Check sheet for the modelled part. Datum: model origin and axes. Units: mm. A direction names the side the tool comes from. Coordinates: 2 decimals unless noted, no trailing zeros. Loops run counter-clockwise (first coordinate to the right, second up) from the corner with the lowest first, then second, coordinate; pieces in that order, holes last. Notation, with made-up numbers: M 38,82 L 78,82 A16 ccw 78,93 Z; hole C 71,-36 d11. An arc over 180 degrees is marked long. Answer as CSV lines item,"result". Start each with the question number.
from build123d import *

# Parameters (mm, degrees)
F1_DEPTH = 15
F2_R     = 10
F3_R     = 5
F4_R     = 5


with BuildPart() as f1:
    # F0 (on Front) → F1 (new body)
    with BuildSketch(Plane.XZ):
        Polygon((41.584589, 20), (41.584589, 0), (48.584589, 0), (48.584589, 27), (19.284589, 27), (19.284589, 7), (-45.715411, 7), (-50.715411, 7), (-50.715411, 0), (26.284589, 0), (26.284589, 20), align=None)
    extrude(amount=F1_DEPTH)

    # F2
    f2_edges = [f1.edges().sort_by_distance(p)[0] for p in [
        (19.284589, -7.5, 7),
    ]]
    fillet(f2_edges, radius=F2_R)

    # F3
    f3_edges = [f1.edges().sort_by_distance(p)[0] for p in [
        (19.284589, -7.5, 27),
    ]]
    fillet(f3_edges, radius=F3_R)

    # F4
    f4_edges = [f1.edges().sort_by_distance(p)[0] for p in [
        (48.584589, -7.5, 27),
    ]]
    fillet(f4_edges, radius=F4_R)


solid = f1.part
Item 1: Go/stop test with flat-tipped pins: pin 1 (4.5 mm diameter, centred on x = -34.5, y = -11, fed in from +Z); pin 2 (1.5 mm diameter, centred on y = -7, z = 19, fed in from -X); pin 3 (7.5 mm diameter, centred on x = 34, y = -8, fed in from -Z). Record where each tip stops, or that it passes through.
Item 2: Sectioned sample at B-B, the plane y = -9. Record the boundary of the cut face in (x, z), and give its area (3 significant figures).
Item 3: Sectioned sample at A-A, the plane z = 4. Record the boundary of the cut face in (x, y).
Item 4: Sectioned sample at C-C, the plane z = 11.5. Record the boundary of the cut face in (x, y), and give its area (3 significant figures).
Item 5: Material ranges on line 1 (X direction, y = -12, z = 2.25); line 2 (X direction, y = -13.75, z = 18.5); line 3 (X direction, y = -6.25, z = 22.25), recorded low to high. Write a range as from..to.
Item 6: Release check for a two-part mould opening along X. For faces 1 (the face through (26.285, -7, 10)), 2 (the face through (34, -7, 27)), 3 (the face through (-50.715, -7, 4)), 4 (the face through (34, -7, 20)) record: released by +X, released by -X, zero draft, split by the parting line, or undercut.
Item 7: Set-up check for faces 5 (the face through (9, 0, 5)), 6 (the face through (-20, -7, 7)), 7 (the face through (41.585, -7, 10)): record each of +Z, -Z, +X, -X, +Y, -Y from which the full face is reachable in a straight line by a thin tool's end or side.
Item 8: Sectioned sample at D-D, the plane x = -2. Record the boundary of the cut face in (y, z), and give its area (3 significant figures).
Reply:
1,pin 1,"z = 7"
1,pin 2,"x = 19.28"
1,pin 3,"z = 20"
2,outline,"M -50.72,0 L 26.28,0 L 26.28,20 L 41.58,20 L 41.58,0 L 48.58,0 L 48.58,22 A5 ccw 43.58,27 L 24.28,27 A5 ccw 19.28,22 L 19.28,17 A10 cw 9.28,7 L -50.72,7 Z"
2,area,"986 mm²"
3,outline,"M -50.72,-15 L 26.28,-15 L 26.28,0 L -50.72,0 Z; M 41.58,-15 L 48.58,-15 L 48.58,0 L 41.58,0 Z"
4,outline,"M 17.64,-15 L 26.28,-15 L 26.28,0 L 17.64,0 Z; M 41.58,-15 L 48.58,-15 L 48.58,0 L 41.58,0 Z"
4,area,"235 mm²"
5,line 1,"-50.72..26.28, 41.58..48.58"
5,line 2,"19.28..26.28, 41.58..48.58"
5,line 3,"19.29..48.58"
6,face 1,"undercut"
6,face 2,"zero draft"
6,face 3,"released by -X"
6,face 4,"undercut"
7,face 5,"+Z, -Z, +X, -X, +Y"
7,face 6,"+Z, -X, +Y, -Y"
7,face 7,"-Z, +Y, -Y"
8,outline,"M -15,0 L 0,0 L 0,7 L -15,7 Z"
8,area,"105 mm²"
